Verification items for the finished model (mm, model axes). A direction names the side the tool comes from. Coordinates: 2 decimals unless noted, no trailing zeros. Order: outer loops, then holes, each group sorted by start corner. A loop starts at its lowest first (then second) coordinate and runs counter-clockwise, first axis right, second up. Notation, with made-up numbers: M 27,68 L 57,68 A15 cw 57,76 Z; hole C 59,68.5 d11. An arc over 180 degrees is marked long. Return JSON: item names as keys, results as strings. Group by question number.
1. Section check B-B, the plane z = 11. Record the cut outline in (x, y), plus the area to 3 significant figures.
2. Section check A-A, the plane y = 25. Give the number of separate pieces and of enclosed holes in the cut face, plus the area to 3 significant figures.
3. Material ranges on line 1 along X through (y, z) = (24, 56); line 2 along Z through (x, y) = (-43.5, 15); line 3 along X through (y, z) = (23.5, 30), recorded low to high.
4. Set-up check for faces 5 (the flat face through (1, 23, -65)), 6 (the flat face through (50.737, 23, -60)), 7 (the flat face through (-51.973, 23, -1)): record each of +Z, -Z, +X, -X, +Y, -Y from which the full face is reachable in a straight line by a thin tool's end or side.
5. Gauge pin test, flat ends, axial feed: pin 1 (0.8 mm diameter, centred on x = -50, y = 15.5, fed in from +Z); pin 2 (0.8 mm diameter, centred on x = 5.5, y = 0, fed in from -Z); pin 3 (2 mm diameter, centred on x = -13.5, z = -13.5, fed in from +Y); pin 4 (4 mm diameter, centred on x = -25.5, z = 21, fed in from -Y). Record the tip position at first contact, or that the pin passes through.
6. Section check D-D, the plane x = -42. Record the cut outline in (y, z), plus the area to 3 significant figures.
7. Section check C-C, the plane x = 28.5. Record the cut outline in (y, z).
8. Mould release check, pull along Z, two halves, no side actions. Record for faces 1 (the flat face through (-50, 23, -60)), 2 (the flat face through (-1, 23, 65.737)), 3 (the flat face through (1, 23, -65.737)), 4 (the flat face through (0.2, 45, -65.5)): +Z half, -Z half, draft (parallel to the pull), parting line (faces both ways), or undercut.
```python
from build123d import *

# Parameters (mm, degrees)
SKETCH1_W                        = 100
SKETCH1_H                        = 130
BASE_FLANGE1_DEPTH               = 0.7366
BOX_REAR_STRIP_W                 = 4.4196
BOX_REAR_STRIP_H                 = 0.7366
BOX_REAR_STRIP_CUT_DEPTH         = 100
BOX_REAR_DEPTH                   = 100
BOX_FRONT_STRIP_W                = 4.4196
BOX_FRONT_STRIP_H                = 0.7366
BOX_FRONT_STRIP_CUT_DEPTH        = 100
BOX_FRONT_DEPTH                  = 100
BOX_FRONT_TABS_STRIP_W           = 4.4196
BOX_FRONT_TABS_STRIP_H           = 0.7366
BOX_FRONT_TABS_STRIP_CUT_DEPTH   = 44.2634
BOX_FRONT_TABS_STRIP_2_W         = 4.4196
BOX_FRONT_TABS_STRIP_2_H         = 0.7366
BOX_FRONT_TABS_STRIP_CUT_2_DEPTH = 44.2634
BOX_FRONT_TABS_DEPTH             = 44.2634
BOX_FRONT_TABS_BEND_DEPTH        = 44.2634
BOX_REAR_TABS_STRIP_W            = 4.4196
BOX_REAR_TABS_STRIP_H            = 0.7366
BOX_REAR_TABS_STRIP_CUT_DEPTH    = 44.2634
BOX_REAR_TABS_STRIP_2_W          = 4.4196
BOX_REAR_TABS_STRIP_2_H          = 0.7366
BOX_REAR_TABS_STRIP_CUT_2_DEPTH  = 44.2634
BOX_REAR_TABS_DEPTH              = 44.2634
BOX_REAR_TABS_BEND_DEPTH         = 44.2634
EDGE_FLANGE6_DEPTH               = 128.5268
EDGE_FLANGE6_START               = 0.7366
EDGE_FLANGE6_FLAT_DEPTH          = 0.7366
EDGE_FLANGE6_BEND_DEPTH          = 128.5268
EDGE_FLANGE6_FLAT_2_DEPTH        = 0.7366


# Sheet-metal steps are written as plain solids
with BuildPart() as part:
    # Sketch1 → Base-Flange1 (new body)
    with BuildSketch(Plane(origin=(0, 0, 0), x_dir=(1, 0, 0), z_dir=(0, 1, 0))):
        Rectangle(SKETCH1_W, SKETCH1_H)
        Polygon((1.25, 30), (7.25, 30), (7.25, -30), (1.25, -30), (1.25, -4), (-3.75, -4), (-3.75, 4), (1.25, 4), align=None, mode=Mode.SUBTRACT)
        Polygon((30.25, 30), (36.25, 30), (36.25, -30), (30.25, -30), (30.25, -4), (25.25, -4), (25.25, 4), (30.25, 4), align=None, mode=Mode.SUBTRACT)
        Polygon((-27.75, 30), (-21.75, 30), (-21.75, -30), (-27.75, -30), (-27.75, -4), (-32.75, -4), (-32.75, 4), (-27.75, 4), align=None, mode=Mode.SUBTRACT)
    extrude(amount=-BASE_FLANGE1_DEPTH)

    # Box rear strip (across the edge) → Box rear strip cut (cut)
    with BuildSketch(Plane(origin=(50, 0, -65), x_dir=(0, 0, 1), z_dir=(-1, 0, 0))):
        with Locations((-1.4732, -0.3683)):
            Rectangle(BOX_REAR_STRIP_W, BOX_REAR_STRIP_H)
    extrude(amount=BOX_REAR_STRIP_CUT_DEPTH, mode=Mode.SUBTRACT)

    # Box rear section (across the edge) → Box rear (add)
    with BuildSketch(Plane(origin=(50, 0, -65), x_dir=(0, 0, 1), z_dir=(-1, 0, 0))):
        with BuildLine():
            Line((-0.7366, 0.7366), (-0.7366, 45))
            Line((-0.7366, 45), (0, 45))
            Line((0, 45), (0, 0.7366))
            ThreePointArc((0, 0.7366), (0.215745145, 0.215745145), (0.7366, 0))
            Line((0.7366, 0), (0.7366, -0.7366))
            ThreePointArc((0.7366, -0.7366), (-0.30510971, -0.30510971), (-0.7366, 0.7366))
        make_face()
    extrude(amount=BOX_REAR_DEPTH)

    # Box front strip (across the edge) → Box front strip cut (cut)
    with BuildSketch(Plane(origin=(-50, 0, 65), x_dir=(0, 0, -1), z_dir=(1, 0, 0))):
        with Locations((-1.4732, -0.3683)):
            Rectangle(BOX_FRONT_STRIP_W, BOX_FRONT_STRIP_H)
    extrude(amount=BOX_FRONT_STRIP_CUT_DEPTH, mode=Mode.SUBTRACT)

    # Box front section (across the edge) → Box front (add)
    with BuildSketch(Plane(origin=(-50, 0, 65), x_dir=(0, 0, -1), z_dir=(1, 0, 0))):
        with BuildLine():
            Line((-0.7366, 0.7366), (-0.7366, 45))
            Line((-0.7366, 45), (0, 45))
            Line((0, 45), (0, 0.7366))
            ThreePointArc((0, 0.7366), (0.215745145, 0.215745145), (0.7366, 0))
            Line((0.7366, 0), (0.7366, -0.7366))
            ThreePointArc((0.7366, -0.7366), (-0.30510971, -0.30510971), (-0.7366, 0.7366))
        make_face()
    extrude(amount=BOX_FRONT_DEPTH)

    # Box-front tabs strip (across the edge) → Box-front tabs strip cut (cut)
    with BuildSketch(Plane(origin=(-50, 0.7366, 65), x_dir=(1, 0, 0), z_dir=(0, 1, 0))):
        with Locations((-1.4732, -0.3683)):
            Rectangle(BOX_FRONT_TABS_STRIP_W, BOX_FRONT_TABS_STRIP_H)
    extrude(amount=BOX_FRONT_TABS_STRIP_CUT_DEPTH, mode=Mode.SUBTRACT)

    # Box-front tabs strip 2 (across the edge) → Box-front tabs strip cut 2 (cut)
    with BuildSketch(Plane(origin=(50, 45, 65), x_dir=(-1, 0, 0), z_dir=(0, -1, 0))):
        with Locations((-1.4732, -0.3683)):
            Rectangle(BOX_FRONT_TABS_STRIP_2_W, BOX_FRONT_TABS_STRIP_2_H)
    extrude(amount=BOX_FRONT_TABS_STRIP_CUT_2_DEPTH, mode=Mode.SUBTRACT)

    # Box-front tabs section (across the edge) → Box-front tabs (add)
    with BuildSketch(Plane(origin=(-50, 0.7366, 65), x_dir=(1, 0, 0), z_dir=(0, 1, 0))):
        with BuildLine():
            Line((-0.7366, 0.7366), (-0.7366, 10))
            Line((-0.7366, 10), (0, 10))
            Line((0, 10), (0, 0.7366))
            ThreePointArc((0, 0.7366), (0.215745145, 0.215745145), (0.7366, 0))
            Line((0.7366, 0), (0.7366, -0.7366))
            ThreePointArc((0.7366, -0.7366), (-0.30510971, -0.30510971), (-0.7366, 0.7366))
        make_face()
    extrude(amount=BOX_FRONT_TABS_DEPTH)

    # Box-front tabs section 2 (across the edge) → Box-front tabs bend (add)
    with BuildSketch(Plane(origin=(50, 45, 65), x_dir=(-1, 0, 0), z_dir=(0, -1, 0))):
        with BuildLine():
            Line((-0.7366, 0.7366), (-0.7366, 10))
            Line((-0.7366, 10), (0, 10))
            Line((0, 10), (0, 0.7366))
            ThreePointArc((0, 0.7366), (0.215745145, 0.215745145), (0.7366, 0))
            Line((0.7366, 0), (0.7366, -0.7366))
            ThreePointArc((0.7366, -0.7366), (-0.30510971, -0.30510971), (-0.7366, 0.7366))
        make_face()
    extrude(amount=BOX_FRONT_TABS_BEND_DEPTH)

    # Box-rear tabs strip (across the edge) → Box-rear tabs strip cut (cut)
    with BuildSketch(Plane(origin=(50, 0.7366, -65), x_dir=(-1, 0, 0), z_dir=(0, 1, 0))):
        with Locations((-1.4732, -0.3683)):
            Rectangle(BOX_REAR_TABS_STRIP_W, BOX_REAR_TABS_STRIP_H)
    extrude(amount=BOX_REAR_TABS_STRIP_CUT_DEPTH, mode=Mode.SUBTRACT)

    # Box-rear tabs strip 2 (across the edge) → Box-rear tabs strip cut 2 (cut)
    with BuildSketch(Plane(origin=(-50, 45, -65), x_dir=(1, 0, 0), z_dir=(0, -1, 0))):
        with Locations((-1.4732, -0.3683)):
            Rectangle(BOX_REAR_TABS_STRIP_2_W, BOX_REAR_TABS_STRIP_2_H)
    extrude(amount=BOX_REAR_TABS_STRIP_CUT_2_DEPTH, mode=Mode.SUBTRACT)

    # Box-rear tabs section (across the edge) → Box-rear tabs (add)
    with BuildSketch(Plane(origin=(50, 0.7366, -65), x_dir=(-1, 0, 0), z_dir=(0, 1, 0))):
        with BuildLine():
            Line((-0.7366, 0.7366), (-0.7366, 10))
            Line((-0.7366, 10), (0, 10))
            Line((0, 10), (0, 0.7366))
            ThreePointArc((0, 0.7366), (0.215745145, 0.215745145), (0.7366, 0))
            Line((0.7366, 0), (0.7366, -0.7366))
            ThreePointArc((0.7366, -0.7366), (-0.30510971, -0.30510971), (-0.7366, 0.7366))
        make_face()
    extrude(amount=BOX_REAR_TABS_DEPTH)

    # Box-rear tabs section 2 (across the edge) → Box-rear tabs bend (add)
    with BuildSketch(Plane(origin=(-50, 45, -65), x_dir=(1, 0, 0), z_dir=(0, -1, 0))):
        with BuildLine():
            Line((-0.7366, 0.7366), (-0.7366, 10))
            Line((-0.7366, 10), (0, 10))
            Line((0, 10), (0, 0.7366))
            ThreePointArc((0, 0.7366), (0.215745145, 0.215745145), (0.7366, 0))
            Line((0.7366, 0), (0.7366, -0.7366))
            ThreePointArc((0.7366, -0.7366), (-0.30510971, -0.30510971), (-0.7366, 0.7366))
        make_face()
    extrude(amount=BOX_REAR_TABS_BEND_DEPTH)

    # Edge-Flange6 bend section (across the edge) → Edge-Flange6 (add)
    with BuildSketch(Plane(origin=(-51.2366, 0, -64.2634), x_dir=(1, 0, 0), z_dir=(0, 0, 1))):
        with BuildLine():
            Line((-0.7366, 0.7366), (0, 0.7366))
            ThreePointArc((0, 0.7366), (0.215745145, 0.215745145), (0.7366, 0))
            Line((0.7366, 0), (1.2366, 0))
            Line((1.2366, 0), (1.2366, -0.7366))
            Line((1.2366, -0.7366), (0.7366, -0.7366))
            ThreePointArc((0.7366, -0.7366), (-0.30510971, -0.30510971), (-0.7366, 0.7366))
        make_face()
    extrude(amount=EDGE_FLANGE6_DEPTH)

    # Edge-Flange6 profile (on flange) → Edge-Flange6 flat (add)
    with BuildSketch(Plane.ZY.offset(51.2366).offset(EDGE_FLANGE6_START)):
        Polygon((-64.2634, 45), (-64.2634, 0.7366), (64.2634, 0.7366), (64.2634, 45), (-2.12, 45), align=None)
    extrude(amount=-EDGE_FLANGE6_FLAT_DEPTH)

    # Edge-Flange6 bend section 2 (across the edge) → Edge-Flange6 bend (add)
    with BuildSketch(Plane(origin=(51.2366, 0, 64.2634), x_dir=(-1, 0, 0), z_dir=(0, 0, -1))):
        with BuildLine():
            Line((-0.7366, 0.7366), (0, 0.7366))
            ThreePointArc((0, 0.7366), (0.215745145, 0.215745145), (0.7366, 0))
            Line((0.7366, 0), (1.2366, 0))
            Line((1.2366, 0), (1.2366, -0.7366))
            Line((1.2366, -0.7366), (0.7366, -0.7366))
            ThreePointArc((0.7366, -0.7366), (-0.30510971, -0.30510971), (-0.7366, 0.7366))
        make_face()
    extrude(amount=EDGE_FLANGE6_BEND_DEPTH)

    # Edge-Flange6 profile 2 (on flange) → Edge-Flange6 flat 2 (add)
    with BuildSketch(Plane(origin=(51.2366, 0, 0), x_dir=(0, 0, -1), z_dir=(1, 0, 0)).offset(EDGE_FLANGE6_START)):
        Polygon((-64.2634, 45), (-64.2634, 0.7366), (64.2634, 0.7366), (64.2634, 45), (-2.12, 45), align=None)
    extrude(amount=-EDGE_FLANGE6_FLAT_2_DEPTH)


solid = part.part
```
Answers follow:
{
 "1": {"outline": "M -51.97,0.74 A1.47 ccw -50.5,-0.74 L -27.75,-0.74 L -27.75,0 L -50.5,0 A0.74 cw -51.24,0.74 L -51.24,45 L -51.97,45 Z; M -21.75,-0.74 L 1.25,-0.74 L 1.25,0 L -21.75,0 Z; M 7.25,-0.74 L 30.25,-0.74 L 30.25,0 L 7.25,0 Z; M 36.25,-0.74 L 50.5,-0.74 A1.47 ccw 51.97,0.74 L 51.97,45 L 51.24,45 L 51.24,0.74 A0.74 cw 50.5,0 L 36.25,0 Z", "area": "129 mm^2"},
 "2": {"separate pieces": "4", "enclosed holes": "0", "area": "367 mm^2"},
 "3": {"line 1": "-51.97 to -51.24, -50.74 to -50, 50 to 50.74, 51.24 to 51.97", "line 2": "-65.74 to -65, 65 to 65.74", "line 3": "-51.97 to -51.24, 51.24 to 51.97"},
 "4": {"face 5": "+Y", "face 6": "+Z, -Z, +Y", "face 7": "+Z, -Z, -X, +Y, -Y"},
 "5": {"pin 1": "z = 65.7", "pin 2": "z = -65.7", "pin 3": "y = 0", "pin 4": "through"},
 "6": {"outline": "M -0.74,-64.26 A1.47 ccw 0.74,-65.74 L 45,-65.74 L 45,-65 L 0.74,-65 A0.74 cw 0,-64.26 L 0,64.26 A0.74 cw 0.74,65 L 45,65 L 45,65.74 L 0.74,65.74 A1.47 ccw -0.74,64.26 Z", "area": "162 mm^2"},
 "7": {"outline": "M -0.74,-64.26 A1.47 ccw 0.74,-65.74 L 45,-65.74 L 45,-65 L 0.74,-65 A0.74 cw 0,-64.26 L 0,-4 L -0.74,-4 Z; M -0.74,4 L 0,4 L 0,64.26 A0.74 cw 0.74,65 L 45,65 L 45,65.74 L 0.74,65.74 A1.47 ccw -0.74,64.26 Z"},
 "8": {"face 1": "undercut", "face 2": "+Z half", "face 3": "-Z half", "face 4": "draft"}
}
